Job drawing, mm, ordinate dimensions from the low corner. One solid piece. A direction names the side the tool comes from. Round coordinates to 2 decimals unless told otherwise and drop trailing zeros. Write each loop counter-clockwise with the first axis right and the second up, starting at its lowest first coordinate (ties: lowest second). Pieces come first, ordered by that corner, then holes. Notation, with made-up numbers: (73, 58.25) -> (122, 58.25) arc R11 ccw to (122, 72.25) -> close; hole circle Ø7 at (3, 14.25). An arc over 180 degrees is marked (long way). Use CSV: the item, a comma, the result in double quotes. Start each with the question number.
(1) Drop a flat-ended pin along its axis: pin 1 (0.8 mm diameter, centred on x = 6, y = 1.5, fed in from -Z). Give the stop position or say it passes through.
(2) Saw through at A-A (z = 4.5). Give the cut face in (x, y), plus the area to 3 significant figures.
(3) Which spindle directions (+Z, -Z, +X, -X, +Y, -Y) get a long thin tool onto all of the face, cutting with end or side? Do the marked faces 5 and 6. Say none if no direction does.
(4) Saw through at C-C (y = 2.2). Count the separate pieces of the cut face and the enclosed holes in it, plus the area to 3 significant figures.
(5) Saw through at B-B (x = 1.5). Give the cut face in (y, z).
(6) Probe line 1 (X direction, y = 2.1, z = 10.75); line 2 (Z direction, x = 5.5, y = 2.2). List the from-to ranges inside material, lowest first. Write a range as [from, to].
(7) Two-plate mould, pull along X, no slides. Class the marked faces 1, 2, 3 and 4: released by +X, released by -X, zero draft, split by the parting line, or undercut.
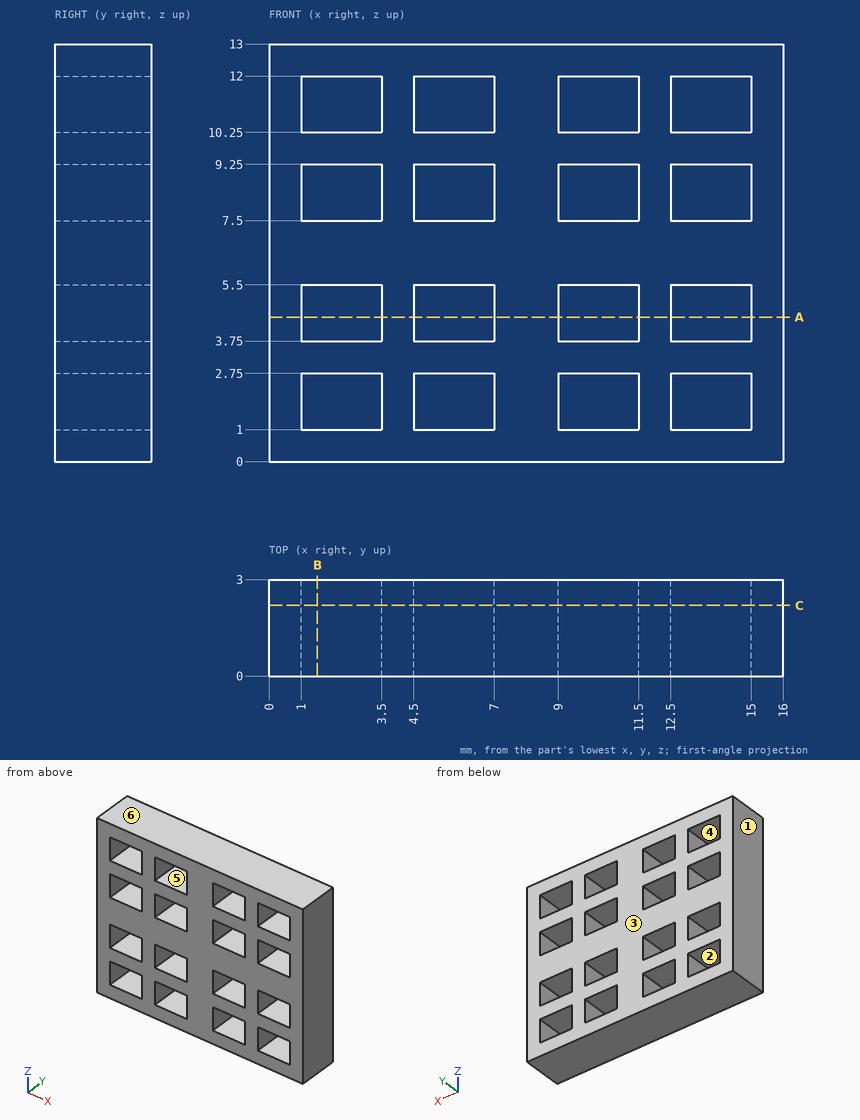
Answers:
1,pin 1,"stops at z = 0"
2,outline,"(0, 0) -> (1, 0) -> (1, 3) -> (0, 3) -> close; (3.5, 0) -> (4.5, 0) -> (4.5, 3) -> (3.5, 3) -> close; (7, 0) -> (9, 0) -> (9, 3) -> (7, 3) -> close; (11.5, 0) -> (12.5, 0) -> (12.5, 3) -> (11.5, 3) -> close; (15, 0) -> (16, 0) -> (16, 3) -> (15, 3) -> close"
2,area,"18.0 mm²"
3,face 5,"+Y, -Y"
3,face 6,"+Z, +X, -X, +Y, -Y"
4,separate pieces,"1"
4,enclosed holes,"16"
4,area,"138 mm²"
5,outline,"(0, 0) -> (3, 0) -> (3, 1) -> (0, 1) -> close; (0, 2.75) -> (3, 2.75) -> (3, 3.75) -> (0, 3.75) -> close; (0, 5.5) -> (3, 5.5) -> (3, 7.5) -> (0, 7.5) -> close; (0, 9.25) -> (3, 9.25) -> (3, 10.25) -> (0, 10.25) -> close; (0, 12) -> (3, 12) -> (3, 13) -> (0, 13) -> close"
6,line 1,"x = [0, 1], [3.5, 4.5], [7, 9], [11.5, 12.5], [15, 16]"
6,line 2,"z = [0, 1], [2.75, 3.75], [5.5, 7.5], [9.25, 10.25], [12, 13]"
7,face 1,"released by -X"
7,face 2,"undercut"
7,face 3,"zero draft"
7,face 4,"undercut"
